The listing builds one solid part. Answer for the finished solid, in the listing's coordinates (mm). A direction names the side the tool comes from. Give positions to 0.01 mm unless a question says otherwise; leave off trailing zeros. Order: outer loops, then holes, each group sorted by start corner. A loop starts at its lowest first (then second) coordinate and runs counter-clockwise, first axis right, second up. Notation, with made-up numbers: (88, 9.5) - (130, 9.5) arc R23 cw to (130, 44.5) - close; hole circle Ø6 at (-16.75, 78). An arc over 180 degrees is marked (long way). Answer in a Markdown table with one row per item. Add a question column.
```python
from build123d import *

# Parameters (mm, degrees)
BOSS_EXTRUDE1_DEPTH = 2
BOSS_EXTRUDE2_DEPTH = 10
CUT_EXTRUDE1_REACH  = 34.605
FILLET1_R           = 2
CHAMFER1_SIZE       = 2


with BuildPart() as part:
    # Sketch1 → Boss-Extrude1 (new body)
    with BuildSketch(Plane(origin=(0, 0, 0), x_dir=(1, 0, 0), z_dir=(0, 1, 0))):
        Polygon((14, 5.75), (-14, 5.75), (-14, -5.75), (-6, -5.75), (-6, -5.25), (-13.5, -5.25), (-13.5, 5.25), (13.5, 5.25), (13.5, -5.25), (6, -5.25), (6, -5.75), (14, -5.75), align=None)
    extrude(amount=BOSS_EXTRUDE1_DEPTH)

    # Sketch2 → Boss-Extrude2 (add)
    with BuildSketch(Plane(origin=(0, 2, 0), x_dir=(1, 0, 0), z_dir=(0, 1, 0))):
        Polygon((-14.8, 6.55), (-14.8, -5.75), (-14, -5.75), (-14, 5.75), (14, 5.75), (14, -5.75), (14.8, -5.75), (14.8, 6.55), align=None)
        Polygon((-14, 5.75), (-14, -5.75), (-6, -5.75), (-6, -5.25), (-13.5, -5.25), (-13.5, 5.25), (13.5, 5.25), (13.5, -5.25), (6, -5.25), (6, -5.75), (14, -5.75), (14, 5.75), align=None)
        Polygon((-6, -5.75), (-5.2, -5.75), (-5.2, -4.45), (-12.7, -4.45), (-12.7, 4.45), (12.7, 4.45), (12.7, -4.45), (5.2, -4.45), (5.2, -5.75), (6, -5.75), (6, -5.25), (13.5, -5.25), (13.5, 5.25), (-13.5, 5.25), (-13.5, -5.25), (-6, -5.25), align=None)
        Polygon((-5.2, -4.45), (-5.2, -5.75), (5.2, -5.75), (5.2, -4.45), (12.7, -4.45), (12.7, 4.45), (-12.7, 4.45), (-12.7, -4.45), align=None)
    extrude(amount=BOSS_EXTRUDE2_DEPTH)

    # Sketch3 → Cut-Extrude1 (cut, up to next)
    with BuildSketch(Plane(origin=(14.8, 0, 0), x_dir=(0, 0, -1), z_dir=(1, 0, 0)), mode=Mode.PRIVATE) as cut_extrude1_sk1:
        with BuildLine():
            Line((6.55, 12), (-3.45, 12))
            ThreePointArc((-3.45, 12), (3.621067812, 9.071067812), (6.55, 2))
            Line((6.55, 2), (6.55, 12))
        make_face()
    cut_extrude1_tool1 = extrude(cut_extrude1_sk1.sketch, amount=-CUT_EXTRUDE1_REACH, mode=Mode.PRIVATE) & part.part
    add(cut_extrude1_tool1.solids().sort_by_distance((14.8, 9.766321, -4.316321))[0], mode=Mode.SUBTRACT)

    # Fillet1
    fillet1_edges = [part.edges().sort_by_distance(p)[0] for p in [
        (14.8, 12, 4.6),
        (-14.8, 12, 4.6),
        (14.8, 9.071067812, -3.621067812),
        (-14.8, 9.071067812, -3.621067812),
    ]]
    fillet(fillet1_edges, radius=FILLET1_R)

    # Chamfer1
    chamfer1_edges = [part.edges().sort_by_distance(p)[0] for p in [
        (0, 2, -5.25),
    ]]
    chamfer(chamfer1_edges, length=CHAMFER1_SIZE - 0.0001)  # a hair under: the kernel refuses the full size


solid = part.part
```
(1) Find section B-B, the plane z = 4.5. Write down the section's boundary in (x, y), plus the area to 3 significant figures.
(2) Straight lines are drawn through the part: line 1 (X direction, y = 0.5, z = -2.75); line 2 (X direction, y = 10.75, z = -0.5); line 3 (Y direction, x = 7.5, z = 4.5). For each, find the intervals that lie inside material, in ascending order.
(3) Find section C-C, the plane y = 1.5. Write down the section's boundary in (x, z).
(4) The mould has two halves that part along Z. Classify faces 4 (the face through (0, 6, 5.75)), 5 (the face through (0, 2, 1)), 6 (the face through (-14, 1, 0)), 7 (the face through (10, 1, 5.25)): +Z half, -Z half, draft (parallel to the pull), parting line (faces both ways), or undercut.
(5) For faces 1 (the face through (14, 1, 0)), 2 (the face through (-10, 1, 5.25)), 3 (the face through (0, 1, -5.75)), determine the directions among +Z, -Z, +X, -X, +Y, -Y from which every point of the face is accessible in a straight line to the end or side of a thin tool.
(6) Each of these flat-tipped pins is pushed along its axis until it touches: P1, Ø0.6, axis at y = 0.5, z = 5.5, coming from the +X side; P2, Ø2, axis at x = -3, z = -0.5, coming from the +Y side (3 decimals); P3, Ø6, axis at x = 5.5, z = -2, coming from the -Y side. Where does it stop, or does it pass through?
Answer key:
| question | item | result |
|---|---|---|
| 1 | outline | (-14.8, 2) - (-14, 2) - (-14, 0) - (-13.5, 0) - (-13.5, 2) - (13.5, 2) - (13.5, 0) - (14, 0) - (14, 2) - (14.8, 2) - (14.8, 10) arc R2 ccw to (12.8, 12) - (-12.8, 12) arc R2 ccw to (-14.8, 10) - close |
| 1 | area | 296 mm² |
| 2 | line 1 | -14 to -13.5, 13.5 to 14 |
| 2 | line 2 | -14 to 14 |
| 2 | line 3 | 2 to 12 |
| 3 | outline | (-14, -5.75) - (14, -5.75) - (14, 5.75) - (6, 5.75) - (6, 5.25) - (13.5, 5.25) - (13.5, -3.75) - (-13.5, -3.75) - (-13.5, 5.25) - (-6, 5.25) - (-6, 5.75) - (-14, 5.75) - close |
| 4 | face 4 | +Z half |
| 4 | face 5 | undercut |
| 4 | face 6 | draft |
| 4 | face 7 | undercut |
| 5 | face 1 | +Z, -Z, +X, -Y |
| 5 | face 2 | -Y |
| 5 | face 3 | -Z, +X, -X, -Y |
| 6 | P1 | x = 14 |
| 6 | P2 | y = 11.555 |
| 6 | P3 | y = 0.25 |
